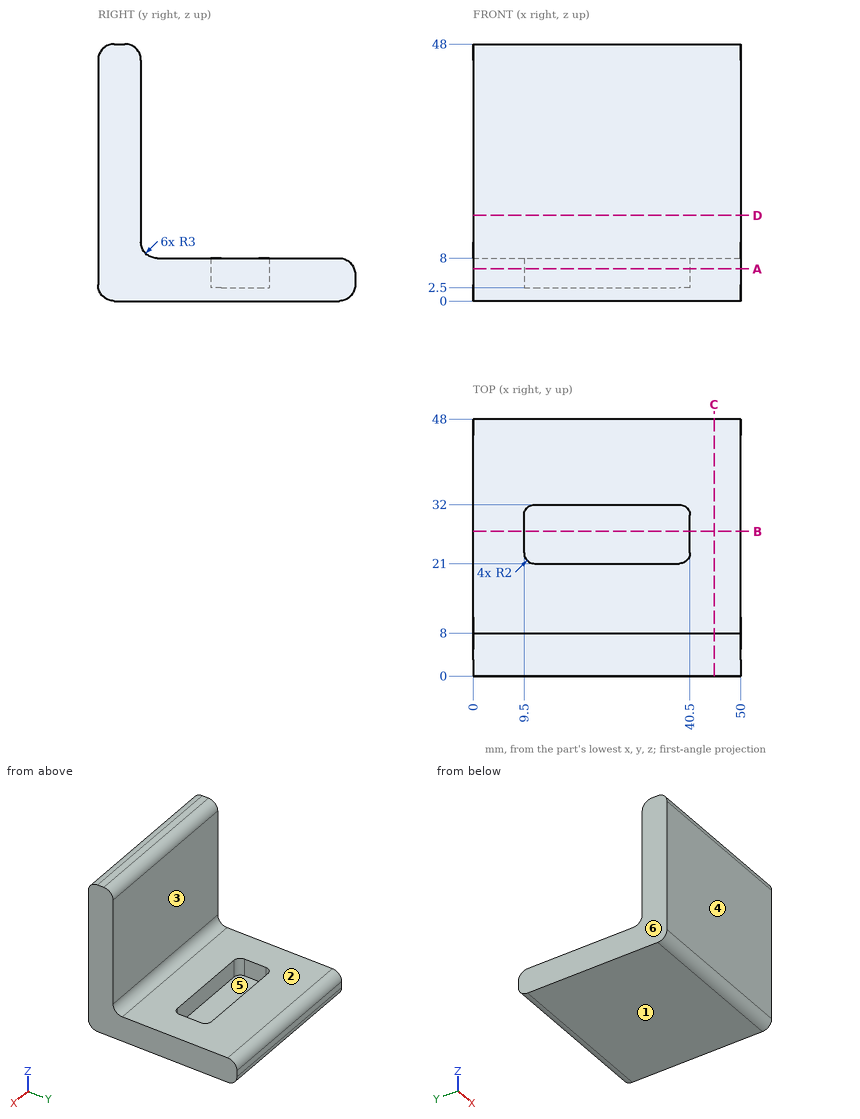
Study the drawing (mm; zero at the part's minimum x, y, z) and answer. A direction names the side the tool comes from. Coordinates: 2 decimals unless noted, no trailing zeros. Loops run counter-clockwise (first coordinate to the right, second up) from the corner with the lowest first, then second, coordinate; pieces in that order, holes last. Notation, with made-up numbers: (-38.75, -34.75) -> (20.25, -34.75) arc R9 ccw to (20.25, -21.75) -> close; hole circle Ø7 at (66.5, 31). An arc over 180 degrees is marked (long way). Answer as CSV lines item,"result".
1) For a pull along Y with two mould halves and no side action, classify the marked faces 3, 4, 5 and 6 as released by +Y, released by -Y, zero draft, split by the parting line, or undercut.
A:
face 3,"released by +Y"
face 4,"released by -Y"
face 5,"undercut"
face 6,"zero draft"
2) Flat-ended cylindrical pins translate along their axes: pin 1 (1 mm diameter, centred on x = 12.5, y = 33, fed in from +Z); pin 2 (5 mm diameter, centred on y = 12.5, z = 12, fed in from -X); pin 3 (17 mm diameter, centred on x = 14.5, z = 32, fed in from +Y). Find the tip coordinate at first contact, or state that the pin passes through.
A:
pin 1,"stops at z = 8"
pin 2,"passes through"
pin 3,"stops at y = 8"
3) The part is cut by section C-C (x = 45). Give the vertices of the cut face in (y, z).
A:
outline,"(0, 3) arc R3 ccw to (3, 0) -> (45, 0) arc R3 ccw to (48, 3) -> (48, 5) arc R3 ccw to (45, 8) -> (11, 8) arc R3 cw to (8, 11) -> (8, 45) arc R3 ccw to (5, 48) -> (3, 48) arc R3 ccw to (0, 45) -> close"
4) Straight lines are drawn through the part: probe 1 along X at (y, z) = (30, 6.5); probe 2 along Z at (x, y) = (18, 35.5). For each, find the intervals that lie inside material, in ascending order.
A:
probe 1,"x = 0 to 9.5, 40.5 to 50"
probe 2,"z = 0 to 8"
5) The part is cut by section D-D (z = 16). Give the vertices of the cut face in (x, y).
A:
outline,"(0, 0) -> (50, 0) -> (50, 8) -> (0, 8) -> close"
6) The part is cut by section A-A (z = 6). Give the vertices of the cut face in (x, y).
A:
outline,"(0, 0) -> (50, 0) -> (50, 47.83) -> (0, 47.83) -> close; hole (9.5, 23) arc R2 ccw to (11.5, 21) -> (38.5, 21) arc R2 ccw to (40.5, 23) -> (40.5, 30) arc R2 ccw to (38.5, 32) -> (11.5, 32) arc R2 ccw to (9.5, 30) -> close"
7) The part is cut by section B-B (y = 27). Give the vertices of the cut face in (x, z).
A:
outline,"(0, 0) -> (50, 0) -> (50, 8) -> (40.5, 8) -> (40.5, 2.5) -> (9.5, 2.5) -> (9.5, 8) -> (0, 8) -> close"
8) For the marked faces 1 and 2, determine the directions among +Z, -Z, +X, -X, +Y, -Y from which every point of the face is accessible in a straight line to the end or side of a thin tool.
A:
face 1,"-Z, +X, -X, +Y, -Y"
face 2,"+Z, +X, -X, +Y"
